Design review of the part built by this model. Coordinates are the model's own, in mm. Give positions to 0.01 mm unless a question says otherwise; leave off trailing zeros. Loops run counter-clockwise (first coordinate to the right, second up) from the corner with the lowest first, then second, coordinate; pieces in that order, holes last. Notation, with made-up numbers: M 21,75 L 65,75 A29 ccw 65,102 Z; hole C 85.25,69.25 d3. An arc over 180 degrees is marked long. Answer as CSV lines item,"result".
```python
from build123d import *

# Parameters (mm, degrees)
SKETCH1_W           = 80
SKETCH1_H           = 30
BOSS_EXTRUDE1_DEPTH = 110
FILLET1_RADIUS      = 40
FILLET1_LENGTH      = 30
FILLET2_R           = 5
CUT_EXTRUDE1_REACH  = 122.83
SKETCH2_R           = 17


with BuildPart() as part:
    # Sketch1 → Boss-Extrude1 (new body)
    with BuildSketch(Plane.XY):
        with Locations((0, 15)):
            Rectangle(SKETCH1_W, SKETCH1_H)
    extrude(amount=BOSS_EXTRUDE1_DEPTH)

    # Fillet1: full round fillet: the end face becomes a half cylinder, R = half its width
    fillet1_face = Plane((0, 15, 110), x_dir=(0, -1, 0), z_dir=(0, 0, 1))  # on the end face: x along it, z out of the body
    fillet1_slab = fillet1_face.offset(-FILLET1_RADIUS / 2) * Box(FILLET1_LENGTH, 2 * FILLET1_RADIUS, FILLET1_RADIUS, mode=Mode.PRIVATE)  # the body's end, R deep
    fillet1_round = Plane((0, 15, 70), x_dir=(0, 0, 1), z_dir=(0, -1, 0)) * Cylinder(FILLET1_RADIUS, FILLET1_LENGTH, mode=Mode.PRIVATE)  # its axis R under the face
    add(fillet1_slab - fillet1_round, mode=Mode.SUBTRACT)

    # Fillet2
    fillet2_edges = [part.edges().sort_by_distance(p)[0] for p in [
        (40, 30, 35),
        (40, 0, 35),
        (-40, 0, 35),
        (-40, 30, 35),
        (0, 30, 110),
        (0, 0, 110),
    ]]
    fillet(fillet2_edges, radius=FILLET2_R)

    # Sketch2 → Cut-Extrude1 (cut, up to next)
    with BuildSketch(Plane.XZ, mode=Mode.PRIVATE) as cut_extrude1_sk1:
        with Locations((0, 70.95)):
            Circle(SKETCH2_R)
    cut_extrude1_tool1 = extrude(cut_extrude1_sk1.sketch, amount=-CUT_EXTRUDE1_REACH, mode=Mode.PRIVATE) & part.part
    add(cut_extrude1_tool1.solids().sort_by_distance((0, 0, 70.95))[0], mode=Mode.SUBTRACT)


solid = part.part
```
1. We need section A-A, the plane x = 0. Write out the cut boundary in (y, z), plus the area to 3 significant figures.
Answer block:
outline,"M 0,0 L 30,0 L 30,53.95 L 0,53.95 Z; M 0,87.95 L 30,87.95 L 30,105 A5 ccw 25,110 L 5,110 A5 ccw 0,105 Z"
area,"2,270 mm²"
2. To check wall thickness, follow L1, parallel to Z at x = 0, y = 18.5; L2, parallel to X at y = 9, z = 68.5; L3, parallel to X at y = 9.75, z = 57.5. State the ranges of each line that lie inside material, in increasing order. Write a range as [from, to].
Answer block:
L1,"[0, 53.95], [87.95, 110]"
L2,"[-40, -16.82], [16.82, 40]"
L3,"[-40, -10.4], [10.4, 40]"
3. For P1, Ø10, axis at x = -21, y = 14, coming from the +Z side; P2, Ø5, axis at y = 8.5, z = 84.5, coming from the -X side; P3, Ø1, axis at x = 26.5, y = 20.5, coming from the +Z side, all flat-tipped, find the tip position at first contact; note any pin that passes through.
Answer block:
P1,"z = 106.66"
P2,"x = -38.16"
P3,"z = 100.4"
4. We need section B-B, the plane y = 16.5. Write out the cut boundary in (x, z).
Answer block:
outline,"M -40,0 L 40,0 L 40,70 A40 ccw -40,70 Z; hole C 0,70.95 d34"
5. We need section C-C, the plane z = 63.5. Write out the cut boundary in (x, y), plus the area to 3 significant figures.
Answer block:
outline,"M -40,5 A5 ccw -35,0 L -15.28,0 L -15.28,30 L -35,30 A5 ccw -40,25 Z; M 15.28,0 L 35,0 A5 ccw 40,5 L 40,25 A5 ccw 35,30 L 15.28,30 Z"
area,"1,460 mm²"
